Here's how the part is built. I have some questions about the finished solid (model axes, mm). Round coordinates to 2 decimals unless told otherwise and drop trailing zeros. Loops run counter-clockwise (first coordinate to the right, second up) from the corner with the lowest first, then second, coordinate; pieces in that order, holes last. Notation, with made-up numbers: (36.25, -39) -> (84.25, -39) arc R23 ccw to (84.25, -2) -> close; hole circle Ø9 at (-40, 41). An arc over 180 degrees is marked (long way). Use one line per item in the form item = value. Start each with the question number.
Item 1: If we section it at B-B (z = 9.75): Write out the boundary of the cut face in (x, y), then the cut area to 3 significant figures.
Item 2: If we section it at A-A (z = 2.5): Write out the boundary of the cut face in (x, y).
Item 3: I'm going to push flat-ended pins straight in: pin 1 Ø1.5 at (x, z) = (6.5, 7) entering from -Y; pin 2 Ø1 at (x, z) = (-1.5, 8) entering from -Y; pin 3 Ø3 at (x, z) = (2.5, 13.5) entering from +Y; pin 4 Ø8 at (x, y) = (3, -2.5) entering from +Z. Where does each tip first touch, or does it pass through?
Item 4: If I drill on L1, parallel to X at y = 6, z = 3.25; L2, parallel to X at y = -8.75, z = 2.75; L3, parallel to Z at x = 6, y = -2.5, over which ranges is the centre line in solid material (lowest first)? Write a range as [from, to].
```python
from build123d import *

# Parameters (mm, degrees)
F2_R = 1.216625
F3_R = 1.031815
F4_R = 1.144544
F5_R = 14.206331
F6_R = 8.725041


with BuildPart() as f1:
    # F0 (on Front) → F1 (revolve)
    with BuildSketch(Plane.XZ):
        Polygon((-10.26025, 0), (0, 0), (0, 15), (-3.757334, 12.255651), (-6.561344, 8.019807), (-5.964746, 7.184571), (-7.39658, 6.945931), (-9.186374, 4.082262), align=None)
    revolve(axis=Axis((0, 0, 7.5), (0, 0, -1)))

    # F2
    f2_edges = [f1.edges().sort_by_distance(p)[0] for p in [
        (6.561344, 0, 8.019807),
    ]]
    fillet(f2_edges, radius=F2_R)

    # F3
    f3_edges = [f1.edges().sort_by_distance(p)[0] for p in [
        (7.39658, 0, 6.945931),
    ]]
    fillet(f3_edges, radius=F3_R)

    # F4
    f4_edges = [f1.edges().sort_by_distance(p)[0] for p in [
        (10.26025, 0, 0),
    ]]
    fillet(f4_edges, radius=F4_R)

    # F5
    f5_edges = [f1.edges().sort_by_distance(p)[0] for p in [
        (3.757334, 0, 12.255651),
    ]]
    fillet(f5_edges, radius=F5_R)

    # F6
    f6_edges = [f1.edges().sort_by_distance(p)[0] for p in [
        (9.186374, 0, 4.082262),
    ]]
    fillet(f6_edges, radius=F6_R)


solid = f1.part
```
Values found:
q1.outline = circle Ø10.83 at (0, 0)
q1.area = 92.2 mm2
q2.outline = circle Ø19.21 at (0, 0)
q3.pin_1 = -4.86
q3.pin_2 = -6.22
q3.pin_3 = 3.03
q3.pin_4 = 15
q4.L1 = [-7.23, 7.23]
q4.L2 = [-3.79, 3.79]
q4.L3 = [0, 7.1]
